```python
from build123d import *

# Parameters (mm, degrees)
SKETCH1_R           = 11.15
BOSS_EXTRUDE1_DEPTH = 15
FILLET1_R           = 0.5


with BuildPart() as part:
    # Sketch1 → Boss-Extrude1 (new body)
    with BuildSketch(Plane(origin=(0, 0, 0), x_dir=(1, 0, 0), z_dir=(0, 1, 0))):
        Polygon((0, 15.55956659), (-1.24854043, 12.676643718), (-3.035520856, 15.260593881), (-3.69764058, 12.189487409), (-5.954388349, 14.375165107), (-6.004642477, 11.233895935), (-8.644432036, 12.9373068), (-8.080889331, 9.84659214), (-11.002275048, 11.002275048), (-9.84659214, 8.080889331), (-12.9373068, 8.644432036), (-11.233895935, 6.004642477), (-14.375165107, 5.954388349), (-12.189487409, 3.69764058), (-15.260593881, 3.035520856), (-12.676643718, 1.24854043), (-15.55956659, 0), (-12.676643718, -1.24854043), (-15.260593881, -3.035520856), (-12.189487409, -3.69764058), (-14.375165107, -5.954388349), (-11.233895935, -6.004642477), (-12.9373068, -8.644432036), (-9.84659214, -8.080889331), (-11.002275048, -11.002275048), (-8.080889331, -9.84659214), (-8.644432036, -12.9373068), (-6.004642477, -11.233895935), (-5.954388349, -14.375165107), (-3.69764058, -12.189487409), (-3.035520856, -15.260593881), (-1.24854043, -12.676643718), (0, -15.55956659), (1.24854043, -12.676643718), (3.035520856, -15.260593881), (3.69764058, -12.189487409), (5.954388349, -14.375165107), (6.004642477, -11.233895935), (8.644432036, -12.9373068), (8.080889331, -9.84659214), (11.002275048, -11.002275048), (9.84659214, -8.080889331), (12.9373068, -8.644432036), (11.233895935, -6.004642477), (14.375165107, -5.954388349), (12.189487409, -3.69764058), (15.260593881, -3.035520856), (12.676643718, -1.24854043), (15.55956659, 0), (12.676643718, 1.24854043), (15.260593881, 3.035520856), (12.189487409, 3.69764058), (14.375165107, 5.954388349), (11.233895935, 6.004642477), (12.9373068, 8.644432036), (9.84659214, 8.080889331), (11.002275048, 11.002275048), (8.080889331, 9.84659214), (8.644432036, 12.9373068), (6.004642477, 11.233895935), (5.954388349, 14.375165107), (3.69764058, 12.189487409), (3.035520856, 15.260593881), (1.24854043, 12.676643718), align=None)
        Circle(SKETCH1_R, mode=Mode.SUBTRACT)
    extrude(amount=BOSS_EXTRUDE1_DEPTH)

    # Fillet1
    fillet1_edges = [part.edges().sort_by_distance(p)[0] for p in [
        (0, 7.5, -15.55956659),
        (3.035520856, 7.5, -15.260593881),
        (5.954388349, 7.5, -14.375165107),
        (8.644432036, 7.5, -12.9373068),
        (11.002275048, 7.5, -11.002275048),
        (12.9373068, 7.5, -8.644432036),
        (14.375165107, 7.5, -5.954388349),
        (15.260593881, 7.5, -3.035520856),
        (15.55956659, 7.5, 0),
        (15.260593881, 7.5, 3.035520856),
        (14.375165107, 7.5, 5.954388349),
        (12.9373068, 7.5, 8.644432036),
        (11.002275048, 7.5, 11.002275048),
        (8.644432036, 7.5, 12.9373068),
        (5.954388349, 7.5, 14.375165107),
        (3.035520856, 7.5, 15.260593881),
        (0, 7.5, 15.55956659),
        (-3.035520856, 7.5, 15.260593881),
        (-5.954388349, 7.5, 14.375165107),
        (-8.644432036, 7.5, 12.9373068),
        (-11.002275048, 7.5, 11.002275048),
        (-12.9373068, 7.5, 8.644432036),
        (-14.375165107, 7.5, 5.954388349),
        (-15.260593881, 7.5, 3.035520856),
        (-15.55956659, 7.5, 0),
        (-15.260593881, 7.5, -3.035520856),
        (-14.375165107, 7.5, -5.954388349),
        (-12.9373068, 7.5, -8.644432036),
        (-11.002275048, 7.5, -11.002275048),
        (-8.644432036, 7.5, -12.9373068),
        (-5.954388349, 7.5, -14.375165107),
        (-3.035520856, 7.5, -15.260593881),
    ]]
    fillet(fillet1_edges, radius=FILLET1_R)


solid = part.part
```
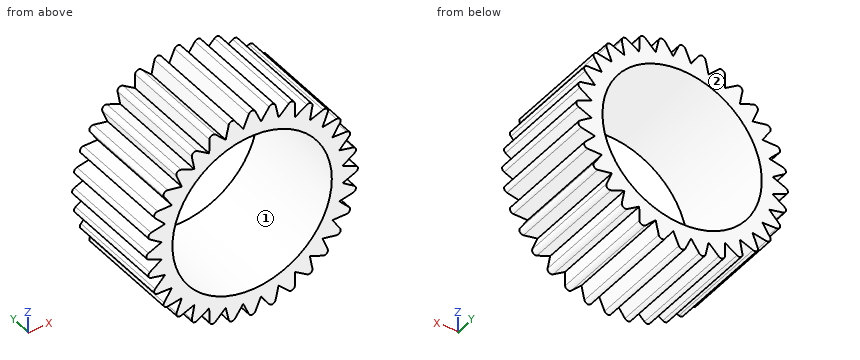
The listing builds one solid part. Answer for the finished solid, in the listing's coordinates (mm). Face numbers are marked on the shaded views. Give positions to 0.01 mm unless a question says otherwise; leave off trailing zeros. Order: outer loops, then holes, each group sorted by start corner. A loop starts at its lowest first (then second) coordinate and runs counter-clockwise, first axis right, second up.
Item 1: Given pin 1 Ø5 at (x, y) = (-6.5, 10.5) entering from +Z; pin 2 Ø6 at (x, y) = (0.5, 12) entering from +Z; pin 3 Ø8 at (y, z) = (7, -8) entering from -X, each flat-ended and moving along its own axis, determine where each tip first touches the part or whether it passes through.
From the geometry:
pin 1: stops at z = 13.71
pin 2: stops at z = 14.8
pin 3: stops at x = -13.71
Item 2: Find the intervals of material crossed by probe 1 along X at (y, z) = (8.5, 0); probe 2 along Z at (x, y) = (-12, 10.75); probe 3 along X at (y, z) = (0.75, -13.5), in increasing order.
From the geometry:
probe 1: x = -14.8 to -11.15, 11.15 to 14.8
probe 2: z = -8.43 to -7.19, -5.99 to 5.99, 7.19 to 8.43
probe 3: x = -5.88 to -5.05, -3.42 to -1.82, -0.89 to 0.89, 1.82 to 3.42, 5.05 to 5.88
Item 3: For a pull along Z with two mould halves and no side action, classify the marked faces 1 and 2 as pulls with the +Z half, pulls with the -Z half, needs draft (parallel to the pull), parting line crosses it, or undercut.
From the geometry:
face 1: undercut
face 2: needs draft
Item 4: The part is cut by section A-A, the plane z = 0. Give the vertices of the cut face in (x, y), and give its area (3 significant figures).
From the geometry:
outline: (-14.8, 0) - (-11.15, 0) - (-11.15, 15) - (-14.8, 15) - close; (11.15, 0) - (14.8, 0) - (14.8, 15) - (11.15, 15) - close
area: 110 mm2
Item 5: The part is cut by section B-B, the plane x = -7.25. Give the vertices of the cut face in (y, z).
From the geometry:
outline: (0, -12.04) - (15, -12.04) - (15, -8.47) - (0, -8.47) - close; (0, 8.47) - (15, 8.47) - (15, 12.04) - (0, 12.04) - close
